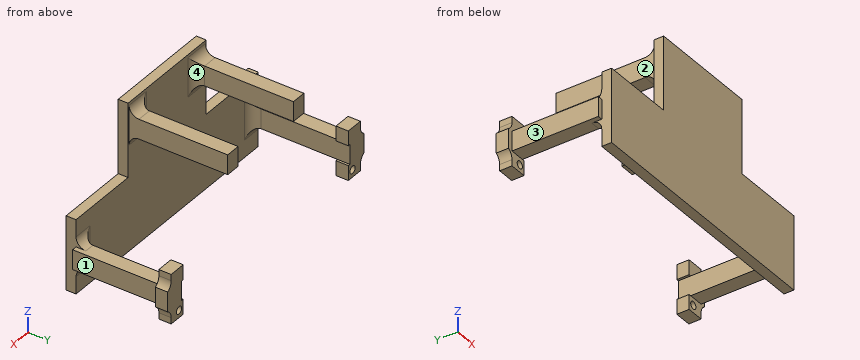
from build123d import *

# Parameters (mm, degrees)
SKETCH1_W            = 45
SKETCH1_H            = 30
BOSS_EXTRUDE1_DEPTH  = 4
SKETCH2_W            = 6
SKETCH2_H            = 8
BOSS_EXTRUDE2_DEPTH  = 40
SKETCH3_W            = 6.928859687
SKETCH3_H            = 6
SKETCH3_R            = 1.5
SKETCH3_W_2          = 2
SKETCH3_H_2          = 8
BOSS_EXTRUDE3_DEPTH  = 5
FILLET2_R            = 4
FILLET3_R            = 4
FILLET2_OF_MIRROR2_R = 4
FILLET3_OF_MIRROR2_R = 4


with BuildPart() as part:
    # Sketch1 → Boss-Extrude1 (new body)
    with BuildSketch(Plane(origin=(0, 0, 0), x_dir=(1, 0, 0), z_dir=(0, 1, 0))):
        Polygon((-22.5, -15), (22.5, -15), (52.5, -15), (52.5, 15), (-52.5, 15), (-52.5, -15), align=None)
        with Locations((0, -30)):
            Rectangle(SKETCH1_W, SKETCH1_H)
    extrude(amount=BOSS_EXTRUDE1_DEPTH)

    # Sketch2 → Boss-Extrude2 (add)
    with BuildSketch(Plane(origin=(0, 4, 0), x_dir=(1, 0, 0), z_dir=(0, 1, 0))):
        with Locations((-51.5, 0)):
            Rectangle(SKETCH2_W, SKETCH2_H)
        with Locations((-18.923893187, -35.779603492)):
            Rectangle(SKETCH2_W, SKETCH2_H)
    boss_extrude2 = extrude(amount=BOSS_EXTRUDE2_DEPTH)

    # Sketch3 → Boss-Extrude3 (add)
    # profile 1 of 3: a face of its own
    with BuildSketch(Plane(origin=(0, 44, 0), x_dir=(1, 0, 0), z_dir=(0, 1, 0))):
        with Locations((-51.035570157, 7)):
            Rectangle(SKETCH3_W, SKETCH3_H)
        with Locations(Location((-50, 7, 0), (0, 0, 270))):
            Circle(SKETCH3_R, mode=Mode.SUBTRACT)
    # profile 2 of 3: a face of its own
    with BuildSketch(Plane(origin=(0, 44, 0), x_dir=(1, 0, 0), z_dir=(0, 1, 0))):
        with Locations((-55.5, 0)):
            Rectangle(SKETCH3_W_2, SKETCH3_H_2)
    # profile 3 of 3: a face of its own
    with BuildSketch(Plane(origin=(0, 44, 0), x_dir=(1, 0, 0), z_dir=(0, 1, 0))):
        with Locations((-51.035570157, -7)):
            Rectangle(SKETCH3_W, SKETCH3_H)
    boss_extrude3 = extrude(amount=-BOSS_EXTRUDE3_DEPTH)

    # Fillet2
    # the kernel refuses this fillet: 4 mm, written as the material it adds along each edge
    with BuildSketch(Plane(origin=(-54.5, 39, -4), x_dir=(0, 0, -1), z_dir=(0, 1, 0))) as fillet2_piece_1:
        with BuildLine():
            CenterArc((3.464101615, 4), FILLET2_R, 210, 60)
            Line((0, 2), (-0.069282032, 1.96))
            ThreePointArc((-0.069282032, 1.96), (-0.08, 1), (-0.08, 0))
            Line((-0.08, 0), (0, -0.08))
            Line((0, -0.08), (3.464101615, -0.08))
            Line((3.464101615, -0.08), (3.464101615, 0))
        make_face()
    extrude(amount=5)
    with BuildSketch(Plane(origin=(-54.5, 39, 4), x_dir=(0, 0, 1), z_dir=(0, 1, 0))) as fillet2_piece_2:
        with BuildLine():
            CenterArc((3.464101615, -4), FILLET2_R, 90, 60)
            Line((0, -2), (-0.069282032, -1.96))
            ThreePointArc((-0.069282032, -1.96), (-0.08, -1), (-0.08, 0))
            Line((-0.08, 0), (0, 0.08))
            Line((0, 0.08), (3.464101615, 0.08))
            Line((3.464101615, 0.08), (3.464101615, 0))
        make_face()
    extrude(amount=5)

    # Fillet3
    fillet3_edges = [part.edges().sort_by_distance(p)[0] for p in [
        (-50.5, 4, 4),
        (-48.5, 4, 0),
        (-50.5, 4, -4),
        (-15.923893187, 4, 35.779603492),
        (-18.923893187, 4, 31.779603492),
        (-18.923893187, 4, 39.779603492),
    ]]
    fillet(fillet3_edges, radius=FILLET3_R)

    # Mirror2: Boss-Extrude2, Boss-Extrude3 across plane
    add(boss_extrude2.mirror(Plane(origin=(0, 0, 0), x_dir=(0, 0, 1), z_dir=(1, 0, 0))))
    add(boss_extrude3.mirror(Plane(origin=(0, 0, 0), x_dir=(0, 0, 1), z_dir=(1, 0, 0))))

    # Fillet2 of Mirror2
    # the kernel refuses this fillet: 4 mm, written as the material it adds along each edge
    with BuildSketch(Plane(origin=(54.5, 39, -4), x_dir=(0, 0, -1), z_dir=(0, 1, 0))) as fillet2_of_mirror2_piece_1:
        with BuildLine():
            CenterArc((3.464101615, -4), FILLET2_OF_MIRROR2_R, 90, 60)
            Line((0, -2), (-0.069282032, -1.96))
            ThreePointArc((-0.069282032, -1.96), (-0.08, -1), (-0.08, 0))
            Line((-0.08, 0), (0, 0.08))
            Line((0, 0.08), (3.464101615, 0.08))
            Line((3.464101615, 0.08), (3.464101615, 0))
        make_face()
    extrude(amount=5)
    with BuildSketch(Plane(origin=(54.5, 39, 4), x_dir=(0, 0, 1), z_dir=(0, 1, 0))) as fillet2_of_mirror2_piece_2:
        with BuildLine():
            CenterArc((3.464101615, 4), FILLET2_OF_MIRROR2_R, 210, 60)
            Line((0, 2), (-0.069282032, 1.96))
            ThreePointArc((-0.069282032, 1.96), (-0.08, 1), (-0.08, 0))
            Line((-0.08, 0), (0, -0.08))
            Line((0, -0.08), (3.464101615, -0.08))
            Line((3.464101615, -0.08), (3.464101615, 0))
        make_face()
    extrude(amount=5)

    # Fillet3 of Mirror2
    fillet3_of_mirror2_edges = [part.edges().sort_by_distance(p)[0] for p in [
        (50.5, 4, 4),
        (48.5, 4, 0),
        (50.5, 4, -4),
        (15.923893187, 4, 35.779603492),
        (18.923893187, 4, 31.779603492),
        (18.923893187, 4, 39.779603492),
    ]]
    fillet(fillet3_of_mirror2_edges, radius=FILLET3_OF_MIRROR2_R)


solid = part.part
Design review of the part built by this model. Coordinates are the model's own, in mm. Face numbers are marked on the shaded views. A direction names the side the tool comes from. Round coordinates to 2 decimals unless told otherwise and drop trailing zeros. Write each loop counter-clockwise with the first axis right and the second up, starting at its lowest first coordinate (ties: lowest second). Pieces come first, ordered by that corner, then holes. Notation, with made-up numbers: (28.25, 8.25) - (61.25, 8.25) arc R25 cw to (61.25, 26.25) - close; hole circle Ø4 at (17.5, 14.5). An arc over 180 degrees is marked (long way). Use a Markdown table: item, result. Add a question column.
1. Wall thickness on probe 1 along X at (y, z) = (41.4, -7); probe 2 along Z at (x, y) = (50, 41.95); probe 3 along Y at (x, z) = (13.5, 8): over which ranges is each line inside the solid? List them lowest first.
2. Clearance check with flat-ended pins moving along their axes: pin 1 (4 mm diameter, centred on x = -50.5, y = 40.5, fed in from +Z); pin 2 (6.5 mm diameter, centred on y = 30, z = 35, fed in from -X); pin 3 (0.7 mm diameter, centred on x = 48, y = 42, fed in from -Z). State where each tip first meets the part, or that it passes through.
3. We need section D-D (z = 13). State the section outline as (x, y) points, then the cut area to 3 significant figures.
4. We need section B-B (y = 23). State the section outline as (x, z) points.
5. We need section C-C (x = 7.5). State the section outline as (y, z) points, then the cut area to 3 significant figures.
6. For the marked faces 1, 2, 3 and 4, list the 3-axis set-ups (+Z, -Z, +X, -X, +Y, -Y) from which the entire face can be reached by the end or side of a thin tool; tool diameter is ignored.
7. We need section A-A (x = 50). State the section outline as (y, z) points.
Output:
| question | item | result |
|---|---|---|
| 1 | probe 1 | x = -54.53 to -51.5, -48.5 to -47.57, 47.57 to 48.5, 51.5 to 54.53 |
| 1 | probe 2 | z = -10 to -8.5, -5.5 to 10 |
| 1 | probe 3 | y = 0 to 4 |
| 2 | pin 1 | stops at z = 10 |
| 2 | pin 2 | stops at x = -21.92 |
| 2 | pin 3 | stops at z = -10 |
| 3 | outline | (-52.5, 0) - (52.5, 0) - (52.5, 4) - (-52.5, 4) - close |
| 3 | area | 420 mm2 |
| 4 | outline | (-54.5, -4) - (-48.5, -4) - (-48.5, 4) - (-54.5, 4) - close; (-21.92, 31.78) - (-15.92, 31.78) - (-15.92, 39.78) - (-21.92, 39.78) - close; (15.92, 31.78) - (21.92, 31.78) - (21.92, 39.78) - (15.92, 39.78) - close; (48.5, -4) - (54.5, -4) - (54.5, 4) - (48.5, 4) - close |
| 5 | outline | (0, -15) - (4, -15) - (4, 45) - (0, 45) - close |
| 5 | area | 240 mm2 |
| 6 | face 1 | +Z, -Z, +X, -Y |
| 6 | face 2 | +Z, -Z, -X, +Y |
| 6 | face 3 | +Z, -Z, -X, -Y |
| 6 | face 4 | +Z, -Z, +Y |
| 7 | outline | (0, -15) - (4, -15) - (4, -8) arc R4 cw to (8, -4) - (39, -4) - (39, -5.5) - (44, -5.5) - (44, 10) - (39, 10) - (39, 4) - (8, 4) arc R4 cw to (4, 8) - (4, 15) - (0, 15) - close; (39, -10) - (44, -10) - (44, -8.5) - (39, -8.5) - close |
